CAD build for the part. Positions are in the model's coordinates, mm. A direction names the side the tool comes from. Round coordinates to 2 decimals unless told otherwise and drop trailing zeros. Write each loop counter-clockwise with the first axis right and the second up, starting at its lowest first coordinate (ties: lowest second). Pieces come first, ordered by that corner, then holes. Notation, with made-up numbers: M 65,58 L 81,58 A21 ccw 81,82 Z; hole C 57,-28 d7. An arc over 180 degrees is marked long. Write each question's results on one line, items separated by ' | '. Start each with the question number.
```python
from build123d import *

# Parameters (mm, degrees)
SKETCH1_W             = 90
SKETCH1_H             = 90
BOSS_EXTRUDE1_DEPTH   = 6.35
F_6_CLEARANCE_HOLE1_D = 3.6576
LPATTERN1_COUNT       = 2
LPATTERN1_PITCH       = 34.925
LPATTERN1_COUNT_DIR2  = 2
LPATTERN1_PITCH_DIR2  = 9.525
F_8_CLEARANCE_HOLE1_D = 4.3053
SKETCH7_W             = 6.35
SKETCH7_H             = 15
CUT_EXTRUDE1_DEPTH    = 64.95562915
F_6_CLEARANCE_HOLE2_D = 3.6576
CUT_EXTRUDE2_DEPTH    = 64.95562915
CUT_EXTRUDE3_DEPTH    = 64.95562915


with BuildPart() as part:
    # Sketch1 → Boss-Extrude1 (new body)
    with BuildSketch(Plane(origin=(0, 0, 0), x_dir=(1, 0, 0), z_dir=(0, 1, 0))):
        Rectangle(SKETCH1_W, SKETCH1_H)
    extrude(amount=BOSS_EXTRUDE1_DEPTH)

    # #6 Clearance Hole1 (through all)
    with Locations(Plane(origin=(0, 6.35, 0), x_dir=(1, 0, 0), z_dir=(0, 1, 0))):
        with Locations((-40.2375, -40.2375)):
            f_6_clearance_hole1 = Hole(F_6_CLEARANCE_HOLE1_D / 2)

    # LPattern1: 6 Clearance Hole1 2 × 2
    with Locations(*[(j * LPATTERN1_PITCH_DIR2, 0, -i * LPATTERN1_PITCH) for i in range(LPATTERN1_COUNT) for j in range(LPATTERN1_COUNT_DIR2) if (i, j) != (0, 0)]):
        add(f_6_clearance_hole1, mode=Mode.SUBTRACT)

    # #8 Clearance Hole1 (through all)
    with Locations(Plane(origin=(0, 6.35, 0), x_dir=(1, 0, 0), z_dir=(0, 1, 0))):
        with Locations((-25, 27.675), (15, 27.675)):
            Hole(F_8_CLEARANCE_HOLE1_D / 2)

    # Sketch7 → Cut-Extrude1 (cut, through all)
    with BuildSketch(Plane(origin=(0, 6.35, 0), x_dir=(1, 0, 0), z_dir=(0, 1, 0))):
        with Locations((3.175, -22.5)):
            Rectangle(SKETCH7_W, SKETCH7_H)
        with Locations((3.175, 22.5)):
            Rectangle(SKETCH7_W, SKETCH7_H)
        with Locations((41.825, -22.5)):
            Rectangle(SKETCH7_W, SKETCH7_H)
        with Locations((41.825, 22.5)):
            Rectangle(SKETCH7_W, SKETCH7_H)
    extrude(amount=-CUT_EXTRUDE1_DEPTH, mode=Mode.SUBTRACT)

    # #6 Clearance Hole2 (through all)
    with Locations(Plane(origin=(0, 6.35, 0), x_dir=(1, 0, 0), z_dir=(0, 1, 0))):
        with Locations((41.825, 0), (3.175, 0)):
            Hole(F_6_CLEARANCE_HOLE2_D / 2)

    # Sketch10 → Cut-Extrude2 (cut, through all)
    with BuildSketch(Plane(origin=(0, 6.35, 0), x_dir=(1, 0, 0), z_dir=(0, 1, 0))):
        Polygon((28.871, -20.60135), (28.871, -24.39865), (32.3714375, -24.39865), (32.3714375, -26.46875), (35.1495625, -26.46875), (35.1495625, -24.39865), (38.65, -24.39865), (38.65, -20.60135), (35.1495625, -20.60135), (35.1495625, -18.53125), (32.3714375, -18.53125), (32.3714375, -20.60135), align=None)
        Polygon((38.65, 24.39865), (38.65, 20.60135), (35.1495625, 20.60135), (35.1495625, 18.53125), (32.3714375, 18.53125), (32.3714375, 20.60135), (28.871, 20.60135), (28.871, 24.39865), (32.3714375, 24.39865), (32.3714375, 26.46875), (35.1495625, 26.46875), (35.1495625, 24.39865), align=None)
    extrude(amount=-CUT_EXTRUDE2_DEPTH, mode=Mode.SUBTRACT)

    # Sketch11 → Cut-Extrude3 (cut, through all)
    with BuildSketch(Plane(origin=(0, 6.35, 0), x_dir=(1, 0, 0), z_dir=(0, 1, 0))):
        Polygon((-45, 15), (-38.65, 15), (-38.65, 20.60135), (-35.1495625, 20.60135), (-35.1495625, 18.53125), (-32.3714375, 18.53125), (-32.3714375, 20.60135), (-28.871, 20.60135), (-28.871, 24.39865), (-32.3714375, 24.39865), (-32.3714375, 26.46875), (-35.1495625, 26.46875), (-35.1495625, 24.39865), (-38.65, 24.39865), (-38.65, 30), (-45, 30), align=None)
    extrude(amount=-CUT_EXTRUDE3_DEPTH, mode=Mode.SUBTRACT)


solid = part.part
```
1) Saw through at B-B, the plane z = 0. Write the cut outline in (x, y).
2) Saw through at A-A, the plane x = 15. Write the cut outline in (y, z), plus the area to 3 significant figures.
3) 3-axis set-ups, long thin cutter, end or side, ignore diameter. For faces 5 (the face through (0, 3, -22)), 6 (the face through (-42, 3, -30)), 7 (the face through (42, 3, 15)): which of +Z, -Z, +X, -X, +Y, -Y reach the whole face in a straight line?
4) Saw through at C-C, the plane y = 3.25. State how many separate pieces and enclosed holes the cut face has, plus the area to 3 significant figures.
5) Drop flat-ended pins along their axis: pin 1 Ø1.7 at (y, z) = (2.5, -18.5) entering from -X; pin 2 Ø3 at (y, z) = (4.5, -28) entering from +X; pin 3 Ø1.7 at (y, z) = (4, -25.5) entering from +X. Give the stop position or say it passes through.
6) Pull direction X, two halves, no side cores. Call faces 1 (the face through (-45, 3, 15)), 2 (the face through (42, 3, -15)), 3 (the face through (3, 3, 15)), 4 (the face through (38.65, 3, -18)): pulls with the +X half, pulls with the -X half, needs draft (parallel to the pull), parting line crosses it, or undercut.
7) Wall check: line 1 along Z through (x, y) = (29.5, 4.25); line 2 along X through (y, z) = (3.5, 25.5); line 3 along Z through (x, y) = (15, 1.75). Give the ranges that are in metal, low to high. Write a range as from..to.
Filled sheet:
1) outline: M -45,0 L 1.35,0 L 1.35,6.35 L -45,6.35 Z; M 5,0 L 40,0 L 40,6.35 L 5,6.35 Z; M 43.65,0 L 45,0 L 45,6.35 L 43.65,6.35 Z
2) outline: M 0,-45 L 6.35,-45 L 6.35,-29.83 L 0,-29.83 Z; M 0,-25.52 L 6.35,-25.52 L 6.35,45 L 0,45 Z | area: 544 mm^2
3) face 5: +Y, -Y | face 6: -X, +Y, -Y | face 7: +X, +Y, -Y
4) separate pieces: 1 | enclosed holes: 10 | area: 7,390 mm^2
5) pin 1: stops at x = -38.65 | pin 2: stops at x = 38.65 | pin 3: stops at x = 38.65
6) face 1: pulls with the -X half | face 2: needs draft | face 3: undercut | face 4: pulls with the +X half
7) line 1: z = -45..-24.4, -20.6..20.6, 24.4..45 | line 2: x = -45..0, 6.35..32.37, 35.15..38.65 | line 3: z = -45..-29.83, -25.52..45
